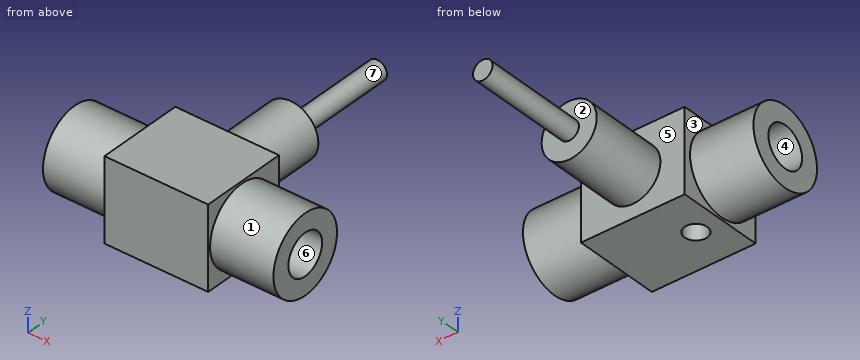
from build123d import *

# Parameters (mm, degrees)
BODY_SKETCH_W                   = 32
BODY_SKETCH_H                   = 26.7
BODY_DEPTH                      = 12.7
NUT_X_SKETCH_W                  = 19.55
NUT_X_SKETCH_H                  = 11.988
NUT_X_SKETCH_2_W                = 19.55
NUT_X_SKETCH_2_H                = 11.988
SOCKET_X_SKETCH_W               = 23.9
SOCKET_X_SKETCH_H               = 6.35
SOCKET_X_SKETCH_2_W             = 23.9
SOCKET_X_SKETCH_2_H             = 6.35
TORCH_NITROUS_PORT_SKETCH_R     = 3.5
TORCH_NITROUS_PORT_DEPTH        = 8.6
TORCH_NITROUS_DRILLING_SKETCH_R = 1
TORCH_NITROUS_DRILLING_DEPTH    = 12.7


with BuildPart() as part:
    # Body Sketch → Body (new, symmetric)
    with BuildSketch(Plane.XY):
        with Locations((0, 0.65)):
            Rectangle(BODY_SKETCH_W, BODY_SKETCH_H)
    extrude(amount=BODY_DEPTH, both=True)

    # Nut _X Sketch → Nut _X (revolve)
    with BuildSketch(Plane.XY, mode=Mode.PRIVATE) as nut_x_sk:
        with Locations((25.775, 5.994)):
            Rectangle(NUT_X_SKETCH_W, NUT_X_SKETCH_H)
    revolve(nut_x_sk.sketch.rotate(Axis((-1000, 0, 0), (1, 0, 0)), 90), axis=Axis((-1000, 0, 0), (1, 0, 0)))

    # Nut -X Sketch 2 → Nut -X 2 (revolve)
    with BuildSketch(Plane.XY, mode=Mode.PRIVATE) as nut_x_2_sk:
        with Locations((-25.775, 5.994)):
            Rectangle(NUT_X_SKETCH_2_W, NUT_X_SKETCH_2_H)
    revolve(nut_x_2_sk.sketch.rotate(Axis((-1000, 0, 0), (1, 0, 0)), 90), axis=Axis((-1000, 0, 0), (1, 0, 0)))

    # Socket _X Sketch → Socket _X (revolve, cut)
    with BuildSketch(Plane.XY, mode=Mode.PRIVATE) as socket_x_sk:
        with Locations((24.6, 3.175)):
            Rectangle(SOCKET_X_SKETCH_W, SOCKET_X_SKETCH_H)
    revolve(socket_x_sk.sketch.rotate(Axis((-1000, 0, 0), (1, 0, 0)), 90), axis=Axis((-1000, 0, 0), (1, 0, 0)), mode=Mode.SUBTRACT)

    # Socket -X Sketch 2 → Socket -X 2 (revolve, cut)
    with BuildSketch(Plane.XY, mode=Mode.PRIVATE) as socket_x_2_sk:
        with Locations((-24.6, 3.175)):
            Rectangle(SOCKET_X_SKETCH_2_W, SOCKET_X_SKETCH_2_H)
    revolve(socket_x_2_sk.sketch.rotate(Axis((-1000, 0, 0), (1, 0, 0)), 90), axis=Axis((-1000, 0, 0), (1, 0, 0)), mode=Mode.SUBTRACT)

    # Stem Sketch → Stem (revolve)
    with BuildSketch(Plane.XY, mode=Mode.PRIVATE) as stem_sk:
        Polygon((0, 14), (8.5, 14), (8.5, 38), (3, 38), (3, 70.6), (0, 70.6), align=None)
    revolve(stem_sk.sketch.rotate(Axis((0, -500, 0), (0, 1, 0)), 90), axis=Axis((0, -500, 0), (0, 1, 0)))

    # Torch Nitrous Port Sketch → Torch Nitrous Port (cut)
    with BuildSketch(Plane.XY.offset(-12.7)):
        with Locations(Location((-8, 0, 0), (0, 0, 180))):
            Circle(TORCH_NITROUS_PORT_SKETCH_R)
    extrude(amount=TORCH_NITROUS_PORT_DEPTH, mode=Mode.SUBTRACT)

    # Torch Nitrous Drilling Sketch → Torch Nitrous Drilling (cut)
    with BuildSketch(Plane.XY.offset(-12.7)):
        with Locations((-8, 0)):
            Circle(TORCH_NITROUS_DRILLING_SKETCH_R)
    extrude(amount=TORCH_NITROUS_DRILLING_DEPTH, mode=Mode.SUBTRACT)


solid = part.part
The listing builds one solid part. Answer for the finished solid, in the listing's coordinates (mm). Face numbers are marked on the shaded views. A direction names the side the tool comes from. Give positions to 0.01 mm unless a question says otherwise; leave off trailing zeros. Order: outer loops, then holes, each group sorted by start corner. A loop starts at its lowest first (then second) coordinate and runs counter-clockwise, first axis right, second up. Notation, with made-up numbers: (-22, 16.25) - (-6, 16.25) arc R17 cw to (-6, 33.25) - close; hole circle Ø10 at (89.5, 76). An arc over 180 degrees is marked (long way). Use one line per item in the form item = value.
1) Each of these flat-tipped pins is pushed along its axis until it touches: pin 1 (10 mm diameter, centred on y = 0, z = 0, fed in from +X); pin 2 (14 mm diameter, centred on y = -0.5, z = -2, fed in from +X); pin 3 (1.6 mm diameter, centred on x = -8, y = 0, fed in from -Z); pin 4 (12 mm diameter, centred on x = -25.5, y = -2.5, fed in from -Z). Where does it stop, or does it pass through?
Verdict:
pin_1 = 12.65
pin_2 = 35.55
pin_3 = 0
pin_4 = -11.99
2) Find section A-A on y = 0. Determine the outline of the cut face in (x, z).
Verdict:
outline = (-35.55, -11.99) - (-16, -11.99) - (-16, -12.7) - (-11.5, -12.7) - (-11.5, -4.1) - (-9, -4.1) - (-9, 0) - (-7, 0) - (-7, -4.1) - (-4.5, -4.1) - (-4.5, -12.7) - (16, -12.7) - (16, -11.99) - (35.55, -11.99) - (35.55, -6.35) - (12.65, -6.35) - (12.65, 6.35) - (35.55, 6.35) - (35.55, 11.99) - (16, 11.99) - (16, 12.7) - (-16, 12.7) - (-16, 11.99) - (-35.55, 11.99) - (-35.55, 6.35) - (-12.65, 6.35) - (-12.65, -6.35) - (-35.55, -6.35) - close
3) Consider probe 1 along Y at (x, z) = (23.5, -0.5); probe 2 along X at (y, z) = (0, -2); probe 3 along Y at (x, z) = (-8, -8.75). Determine where each line is inside the solid, lowest interval first. Write a range as [from, to].
Verdict:
probe_1 = [-11.98, -6.33], [6.33, 11.98]
probe_2 = [-12.65, -9], [-7, 12.65]
probe_3 = [-12.7, -3.5], [3.5, 14]
4) Find section B-B on x = 0. Determine the outline of the cut face in (y, z), and give its area (3 significant figures).
Verdict:
outline = (-12.7, -12.7) - (14, -12.7) - (14, -8.5) - (38, -8.5) - (38, -3) - (70.6, -3) - (70.6, 3) - (38, 3) - (38, 8.5) - (14, 8.5) - (14, 12.7) - (-12.7, 12.7) - close
area = 1,280 mm^2
5) Find section C-C on x = 22. Determine the outline of the cut face in (y, z).
Verdict:
outline = circle Ø23.98 at (0, 0); hole circle Ø12.7 at (0, 0)
6) The mould has two halves that part along Y. Classify the marked faces 4, 5, 6 and 7: released by +Y, released by -Y, zero draft, split by the parting line, or undercut.
Verdict:
face_4 = undercut
face_5 = released by +Y
face_6 = undercut
face_7 = zero draft
7) Find section D-D on z = 7.25. Determine the outline of the cut face in (x, y), and give its area (3 significant figures).
Verdict:
outline = (-35.55, -9.55) - (-16, -9.55) - (-16, -12.7) - (16, -12.7) - (16, -9.55) - (35.55, -9.55) - (35.55, 9.55) - (16, 9.55) - (16, 14) - (4.44, 14) - (4.44, 38) - (-4.44, 38) - (-4.44, 14) - (-16, 14) - (-16, 9.55) - (-35.55, 9.55) - close
area = 1,810 mm^2
8) For the marked faces 1, 2 and 3, determine the directions among +Z, -Z, +X, -X, +Y, -Y from which every point of the face is accessible in a straight line to the end or side of a thin tool.
Verdict:
face_1 = +X
face_2 = +Y
face_3 = -X
